Read the model definition and answer for the solid it produces. Units are mm, in the model's axes. Round coordinates to 2 decimals unless told otherwise and drop trailing zeros. Put each result on its own line as item: value. Start each with the question number.
Q1. Section A-A on z = 4 is taken. State how many separate pieces and enclosed holes the cut face has, then the cut area to 3 significant figures.
Q2. Find the intervals of material crossed by line 1 along Y through (x, z) = (41.15, 3.5); line 2 along Y through (x, z) = (19.5, -5.5); line 3 along X through (y, z) = (-294.4, 1.75), in increasing order. Write a range as from..to.
Q3. Each of these flat-tipped pins is pushed along its axis until it touches: pin 1 Ø7.5 at (x, y) = (-73.15, -294.4) entering from -Z; pin 2 Ø6 at (x, y) = (-73.15, -162.8) entering from +Z; pin 3 Ø5.5 at (x, y) = (20, -266) entering from -Z. Where does it stop, or does it pass through?
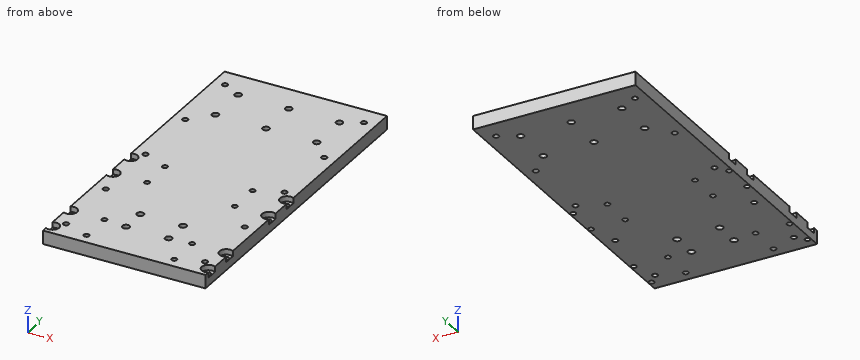
from build123d import *

# Parameters (mm, degrees)
F0_W     = 152.4
F0_H     = 12.7
F1_DEPTH = 304.8
F2_R     = 2.5
F2_R_2   = 3.302
F2_R_3   = 3.175
F2_R_4   = 2.6162
F3_DEPTH = 12.701
F4_R     = 6.35
F5_DEPTH = 5.08


with BuildPart() as f1:
    # F0 (on Front) → F1 (new body)
    with BuildSketch(Plane.XZ):
        Rectangle(F0_W, F0_H)
    extrude(amount=F1_DEPTH)

    # F2 (on face) → F3 (cut, through all)
    with BuildSketch(Plane.XY.offset(6.35)):
        with Locations((-73.15, -294.4)):
            Circle(F2_R)
        with Locations((-41.15, -294.4)):
            Circle(F2_R)
        with Locations((-73.15, -264.4)):
            Circle(F2_R)
        with Locations((-41.15, -264.4)):
            Circle(F2_R)
        with Locations((-73.15, -162.8)):
            Circle(F2_R)
        with Locations((-73.15, -192.8)):
            Circle(F2_R)
        with Locations((-41.15, -192.8)):
            Circle(F2_R)
        with Locations((-41.15, -162.8)):
            Circle(F2_R)
        with Locations((41.15, -162.8)):
            Circle(F2_R)
        with Locations((41.15, -192.8)):
            Circle(F2_R)
        with Locations((73.15, -162.8)):
            Circle(F2_R)
        with Locations((73.15, -192.8)):
            Circle(F2_R)
        with Locations((41.15, -264.4)):
            Circle(F2_R)
        with Locations((73.15, -264.4)):
            Circle(F2_R)
        with Locations((41.15, -294.4)):
            Circle(F2_R)
        with Locations((73.15, -294.4)):
            Circle(F2_R)
        with Locations((-20.0025, -266.0015)):
            Circle(F2_R_2)
        with Locations((-20.0025, -241.9985)):
            Circle(F2_R_2)
        with Locations((20.0025, -241.9985)):
            Circle(F2_R_2)
        with Locations((20.0025, -266.0015)):
            Circle(F2_R_2)
        with Locations((47.5, -28.575)):
            Circle(F2_R_3)
        with Locations((0, -28.575)):
            Circle(F2_R_3)
        with Locations((-47.5, -28.575)):
            Circle(F2_R_3)
        with Locations((-47.5, -66.675)):
            Circle(F2_R_3)
        with Locations((0, -66.675)):
            Circle(F2_R_3)
        with Locations((47.5, -66.675)):
            Circle(F2_R_3)
        with Locations((65.151, -19.05)):
            Circle(F2_R_4)
        with Locations((65.151, -85.725)):
            Circle(F2_R_4)
        with Locations((65.151, -152.4)):
            Circle(F2_R_4)
        with Locations((65.151, -219.075)):
            Circle(F2_R_4)
        with Locations((65.151, -285.75)):
            Circle(F2_R_4)
        with Locations((-65.151, -19.05)):
            Circle(F2_R_4)
        with Locations((-65.151, -85.725)):
            Circle(F2_R_4)
        with Locations((-65.151, -152.4)):
            Circle(F2_R_4)
        with Locations((-65.151, -219.075)):
            Circle(F2_R_4)
        with Locations((-65.151, -285.75)):
            Circle(F2_R_4)
    extrude(amount=-F3_DEPTH, mode=Mode.SUBTRACT)

    # F4 (on face) → F5 (cut)
    with BuildSketch(Plane.XY.offset(6.35)):
        with Locations((-73.15, -294.4)):
            Circle(F4_R)
        with Locations((-73.15, -264.4)):
            Circle(F4_R)
        with Locations((-73.15, -192.8)):
            Circle(F4_R)
        with Locations((-73.15, -162.8)):
            Circle(F4_R)
        with Locations((73.15, -162.8)):
            Circle(F4_R)
        with Locations((73.15, -192.8)):
            Circle(F4_R)
        with Locations((73.15, -264.4)):
            Circle(F4_R)
        with Locations((73.15, -294.4)):
            Circle(F4_R)
    extrude(amount=-F5_DEPTH, mode=Mode.SUBTRACT)


solid = f1.part
Findings:
1. separate pieces: 1
1. enclosed holes: 28
1. area: 44,900 mm2
2. line 1: -304.8..-296.9, -291.9..-266.9, -261.9..-195.3, -190.3..-165.3, -160.3..0
2. line 2: -304.8..-269.27, -262.74..-245.26, -238.73..0
2. line 3: -66.8..-43.65, -38.65..38.65, 43.65..66.8
3. pin 1: z = -6.35
3. pin 2: z = 1.27
3. pin 3: through
